from build123d import *

# Parameters (mm, degrees)
F0_W      = 50.8
F0_H      = 50.8
F1_DEPTH  = 2.9718
F3_W      = 5.08
F3_H      = 50.8
F4_DEPTH  = 2.9728
F2_W      = 5.08
F2_H      = 10.16
F5_DEPTH  = 2.9718
F6_W      = 45.72
F6_H      = 2.2479
F7_DEPTH  = 2.9728
F8_R      = 1.6637
F9_DEPTH  = 2.9728
F10_W     = 10.16
F10_H     = 5.08
F10_R     = 1.6637
F11_DEPTH = 2.9718


with BuildPart() as f1:
    # F0 (on Front) → F1 (new body)
    with BuildSketch(Plane.XZ):
        Rectangle(F0_W, F0_H)
    extrude(amount=F1_DEPTH)

    # F3 (on face) → F4 (cut, through all)
    with BuildSketch(Plane.XZ.offset(2.9718)):
        with Locations((22.86, 0)):
            Rectangle(F3_W, F3_H)
    extrude(amount=-F4_DEPTH, mode=Mode.SUBTRACT)

    # F2 (on face) → F5 (join)
    with BuildSketch(Plane.XZ.offset(2.9718)):
        with Locations((22.745747, 6.871837)):
            Rectangle(F2_W, F2_H)
        with Locations((22.745747, -7.098163)):
            Rectangle(F2_W, F2_H)
    extrude(amount=-F5_DEPTH)

    # F6 (on face) → F7 (cut, through all)
    with BuildSketch(Plane.XZ.offset(2.9718)):
        with Locations((-2.54, -24.27605)):
            Rectangle(F6_W, F6_H)
    extrude(amount=-F7_DEPTH, mode=Mode.SUBTRACT)

    # F8 (on face) → F9 (cut, through all)
    with BuildSketch(Plane.XZ.offset(2.9718)):
        with Locations((22.88278, 6.871837)):
            Circle(F8_R)
        with Locations((22.88278, -7.098163)):
            Circle(F8_R)
    extrude(amount=-F9_DEPTH, mode=Mode.SUBTRACT)

    # F10 (on face) → F11 (join)
    with BuildSketch(Plane.XZ.offset(2.9718)):
        with Locations((-4.13004, -25.6921)):
            Rectangle(F10_W, F10_H)
        with Locations((-4.13004, -25.760639)):
            Circle(F10_R, mode=Mode.SUBTRACT)
    extrude(amount=-F11_DEPTH)


solid = f1.part
Build history of the part. All positions in model axes, mm. A direction names the side the tool comes from. Give positions to 0.01 mm unless a question says otherwise; leave off trailing zeros. Loops run counter-clockwise (first coordinate to the right, second up) from the corner with the lowest first, then second, coordinate; pieces in that order, holes last. Notation, with made-up numbers: (3.5, 85.5) - (10.5, 85.5) arc R27 ccw to (10.5, 116.5) - close; hole circle Ø6 at (-35.75, -31.5). An arc over 180 degrees is marked (long way). Write item = value, one per line. Start each with the question number.
1) Pull direction Z, two halves, no side cores. Call faces 6 (the flat face through (-4, -2, -28.232)), 7 (the flat face through (20.32, -2, 19)), 8 (the cylindrical face through (24.47, -1.51, -6.6)), 9 (the flat face through (-3, -1, 25.4)): +Z half, -Z half, draft (parallel to the pull), parting line (faces both ways), or undercut.
2) Tool access for faces 1 (the flat face through (23, -2, -12.178)), 2 (the flat face through (-9.21, -2, -26)), 3 (the flat face through (23, -2, 1.792)), 4 (the flat face through (0, 0, -1)), 5 (the flat face through (-25.4, -1, 1)): list every direction of +Z, -Z, +X, -X, +Y, -Y with a clear straight run to the whole face (end or side of a thin tool).
3) Probe probe 1 along Z at (x, y) = (-4, -0.3); probe 2 along X at (y, z) = (-2.7, -22.5); probe 3 along Z at (x, y) = (-12.5, -0.4). List the from-to ranges inside material, lowest first. Write a range as from..to.
4) Band-saw the part on D-D on x = -10. Give the cut face in (y, z).
5) Band-saw the part on C-C on z = 15. Give the cut face in (x, y).
6) Band-saw the part on A-A on x = -4.5. Give the cut face in (y, z).
7) Band-saw the part on B-B on x = 22. Give the cut face in (y, z), plus the area to 3 significant figures.
8) Drop flat-ended pins along their axis: pin 1 Ø5.5 at (x, z) = (22.88, 6.87) entering from -Y; pin 2 Ø0.9 at (y, z) = (-1, -15) entering from +X; pin 3 Ø1 at (x, y) = (6, -0.5) entering from -Z; pin 4 Ø2 at (x, z) = (-4.13, -25.76) entering from -Y. Give the stop position or say it passes through.
Final values:
q1.face_6 = -Z half
q1.face_7 = draft
q1.face_8 = undercut
q1.face_9 = +Z half
q2.face_1 = -Z, +X, +Y, -Y
q2.face_2 = -Z, -X, +Y, -Y
q2.face_3 = +X, +Y, -Y
q2.face_4 = +Z, -Z, +X, -X, +Y
q2.face_5 = +Z, -Z, -X, +Y, -Y
q3.probe_1 = -28.23..-27.42, -24.1..25.4
q3.probe_2 = -25.4..20.32
q3.probe_3 = -23.15..25.4
q4.outline = (-2.97, -23.15) - (0, -23.15) - (0, 25.4) - (-2.97, 25.4) - close
q5.outline = (-25.4, -2.97) - (20.32, -2.97) - (20.32, 0) - (-25.4, 0) - close
q6.outline = (-2.97, -28.23) - (0, -28.23) - (0, -27.38) - (-2.97, -27.38) - close; (-2.97, -24.14) - (0, -24.14) - (0, 25.4) - (-2.97, 25.4) - close
q7.outline = (-2.97, -12.18) - (0, -12.18) - (0, -8.51) - (-2.97, -8.51) - close; (-2.97, -5.69) - (0, -5.69) - (0, -2.02) - (-2.97, -2.02) - close; (-2.97, 1.79) - (0, 1.79) - (0, 5.46) - (-2.97, 5.46) - close; (-2.97, 8.28) - (0, 8.28) - (0, 11.95) - (-2.97, 11.95) - close
q7.area = 43.6 mm²
q8.pin_1 = -2.97
q8.pin_2 = 20.32
q8.pin_3 = -23.15
q8.pin_4 = through
